from build123d import *

# Parameters (mm, degrees)
SKETCH3_W           = 25
SKETCH3_H           = 13
BOSS_EXTRUDE1_DEPTH = 8
SKETCH4_W           = 6
SKETCH4_H           = 3.1
CUT_EXTRUDE1_DEPTH  = 5
SKETCH5_W           = 6
SKETCH5_H           = 5
BOSS_EXTRUDE2_DEPTH = 10
CUT_EXTRUDE2_DEPTH  = 10


with BuildPart() as part:
    # Sketch3 → Boss-Extrude1 (new body)
    with BuildSketch(Plane(origin=(0, 0, 0), x_dir=(1, 0, 0), z_dir=(0, 1, 0))):
        with Locations((6.675257732, -1.809278351)):
            Rectangle(SKETCH3_W, SKETCH3_H)
    extrude(amount=BOSS_EXTRUDE1_DEPTH)

    # Sketch4 → Cut-Extrude1 (cut)
    with BuildSketch(Plane.XZ):
        with Locations((6.367389679, 1.844147545)):
            Rectangle(SKETCH4_W, SKETCH4_H)
    extrude(amount=-CUT_EXTRUDE1_DEPTH, mode=Mode.SUBTRACT)

    # Sketch5 → Boss-Extrude2 (add)
    with BuildSketch(Plane(origin=(0, 8, 0), x_dir=(1, 0, 0), z_dir=(0, 1, 0))):
        with Locations((6.675257732, -1.902518117)):
            Rectangle(SKETCH5_W, SKETCH5_H)
    extrude(amount=BOSS_EXTRUDE2_DEPTH)

    # Sketch6 → Cut-Extrude2 (cut)
    with BuildSketch(Plane(origin=(0, 0, -0.597481883), x_dir=(-1, 0, 0), z_dir=(0, 0, -1))):
        with BuildLine():
            Line((-3.675257732, 18), (-6.675257732, 18))
            ThreePointArc((-6.675257732, 18), (-4.610198245, 17.177859086), (-3.675257732, 15.161358998))
            Line((-3.675257732, 15.161358998), (-3.675257732, 18))
        make_face()
        with BuildLine():
            Line((-9.675257732, 18), (-9.675257732, 15.161358998))
            ThreePointArc((-9.675257732, 15.161358998), (-8.740317219, 17.177859086), (-6.675257732, 18))
            Line((-6.675257732, 18), (-9.675257732, 18))
        make_face()
    extrude(amount=-CUT_EXTRUDE2_DEPTH, mode=Mode.SUBTRACT)


solid = part.part
Input: part model. Units: mm. Frame: model coordinates. A direction names the side the tool comes from. Coordinates: 2 decimals unless noted, no trailing zeros. Order: outer loops, then holes, each group sorted by start corner. A loop starts at its lowest first (then second) coordinate and runs counter-clockwise, first axis right, second up. Notation, with made-up numbers: M 49,58 L 83,58 A23 cw 83,88 Z; hole C 64.25,28 d9. An arc over 180 degrees is marked long. Write item = value, one per line. Start each with the question number.
(1) Line query: line 1 along X through (y, z) = (3, 0.5); line 2 along X through (y, z) = (9.75, 0.25); line 3 along Y through (x, z) = (16.5, 4.25). Output: solid intervals per line, ascending. Write a range as [from, to].
(2) Section C-C on y = 14. Output: boundary loops of the cut face in (x, z), and give its area (3 significant figures).
(3) Reachability of faces 1 (the flat face through (9.675, 12, 2)), 2 (the flat face through (7, 13, -0.597)), 3 (the flat face through (3.367, 2, 2)), 4 (the flat face through (3.675, 12, 2)), 5 (the flat face through (7, 13, 4.403)) from +Z, -Z, +X, -X, +Y, -Y: full face, straight path, thin tool, end or side. Return the list, or none.
(4) First-contact query: P1, Ø3, axis at x = 14, z = -3, coming from the +Y side; P2, Ø8, axis at x = 11.5, y = 10, coming from the +Z side; P3, Ø6.5, axis at x = 7.5, y = 11.5, coming from the +Z side; P4, Ø1.5, axis at y = 10.5, z = 1.5, coming from the +X side. Flat tips, straight axial feed; report the tip coordinate or a pass-through.
(5) Section D-D on z = 4. Output: boundary loops of the cut face in (x, y).
(6) Section A-A on z = 1.5. Output: boundary loops of the cut face in (x, y), and give its area (3 significant figures).
(7) Section B-B on x = 8. Output: boundary loops of the cut face in (y, z), and give its area (3 significant figures).
Result set:
q1.line_1 = [-5.82, 3.37], [9.37, 19.18]
q1.line_2 = [3.68, 9.68]
q1.line_3 = [0, 8]
q2.outline = M 3.68,-0.6 L 9.68,-0.6 L 9.68,4.4 L 3.68,4.4 Z
q2.area = 30.0 mm²
q3.face_1 = +Z, -Z, +X, +Y
q3.face_2 = -Z, +X, -X, +Y
q3.face_3 = -Y
q3.face_4 = +Z, -Z, -X, +Y
q3.face_5 = +Z, +X, -X, +Y
q4.P1 = 8
q4.P2 = 8.31
q4.P3 = 4.4
q4.P4 = 9.68
q5.outline = M -5.82,0 L 19.18,0 L 19.18,8 L 9.68,8 L 9.68,15.16 A3 ccw 3.68,15.16 L 3.68,8 L -5.82,8 Z
q6.outline = M -5.82,0 L 3.37,0 L 3.37,5 L 9.37,5 L 9.37,0 L 19.18,0 L 19.18,8 L 9.68,8 L 9.68,15.16 A3 ccw 3.68,15.16 L 3.68,8 L -5.82,8 Z
q6.area = 226 mm²
q7.outline = M 0,-4.69 L 8,-4.69 L 8,-0.6 L 17.69,-0.6 L 17.69,4.4 L 8,4.4 L 8,8.31 L 0,8.31 L 0,3.39 L 5,3.39 L 5,0.29 L 0,0.29 Z
q7.area = 137 mm²
